Read the model definition and answer for the solid it produces. Units are mm, in the model's axes. A direction names the side the tool comes from. Coordinates: 2 decimals unless noted, no trailing zeros. Write each loop counter-clockwise with the first axis right and the second up, starting at its lowest first coordinate (ties: lowest second). Pieces come first, ordered by that corner, then holes. Notation, with made-up numbers: (-9.75, -7.5) -> (13.25, -7.5) arc R26 cw to (13.25, 15.5) -> close; hole circle Ø2 at (60, 23). An arc over 180 degrees is marked (long way). Answer in a Markdown table with one row per item. Add a question column.
Item 1: Section A-A on z = 38 is taken. Write down the section's boundary in (x, y), then the cut area to 3 significant figures.
Item 2: Section B-B on x = -20 is taken. Write down the section's boundary in (y, z).
Item 3: Straight lines are drawn through the part: line 1 (Y direction, x = -20, z = 28.8); line 2 (Y direction, x = 38, z = 28.45); line 3 (Y direction, x = 0, z = 40). For each, find the intervals that lie inside material, in ascending order. Write a range as from..to.
Item 4: Which of the six approach directions +Z, -Z, +X, -X, +Y, -Y give full straight-line access (tool end or side, diameter ignored) to faces 4 (the face through (47.35, 80.07, 37.29)), 5 (the face through (57.45, 61.37, 28.39)), 6 (the face through (10, 34, 28))?
Item 5: Given pin 1 Ø1.6 at (x, y) = (-53, 49.5) entering from +Z; pin 2 Ø1.6 at (y, z) = (34, 28) entering from -X; pin 3 Ø1 at (y, z) = (35, 29) entering from +X; pin 4 Ø10 at (x, y) = (3, 74) entering from +Z, each flat-ended and moving along its own axis, determine where each tip first touches the part or whether it passes through.
Item 6: For a pull along X with two mould halves and no side action, classify faces 1 (the face through (36.85, 40.38, 28.39)), 2 (the face through (58.718, 34.623, 28.386)), 3 (the face through (-46.7, 81.7, 45.4)) as +X half, -X half, draft (parallel to the pull), parting line (faces both ways), or undercut.
Item 7: Section C-C on y = 62 is taken. Write down the section's boundary in (x, z).
Item 8: Section D-D on x = 38 is taken. Write down the section's boundary in (y, z), then the cut area to 3 significant figures.
```python
from build123d import *

# Parameters (mm, degrees)
PAD_DEPTH     = 2
SKETCH001_R   = 3
PAD001_DEPTH  = 16
SKETCH002_R   = 1.6
SKETCH002_R_2 = 1
SKETCH002_R_3 = 1.2
SKETCH002_R_4 = 1.45
POCKET_DEPTH  = 18.001


with BuildPart() as part:
    # Sketch → Pad (new body)
    with BuildSketch(Plane.XY):
        with BuildLine():
            ThreePointArc((-50, 44), (-53.333341, 42.726773), (-54.969042, 39.555534))
            Line((-54.969042, 39.555534), (-60, -5.444466))
            ThreePointArc((-60, -5.444466), (-58.75773, -9.333341), (-55.030958, -11))
            Line((-55.030958, -11), (55.030958, -11))
            ThreePointArc((55.030958, -11), (58.75773, -9.333341), (60, -5.444466))
            Line((54.969042, 39.555534), (60, -5.444466))
            ThreePointArc((54.969042, 39.555534), (53.333341, 42.726773), (50, 44))
            Line((-50, 44), (50, 44))
        make_face()
    extrude(amount=PAD_DEPTH)

    # Sketch001 → Pad001 (join)
    with BuildSketch(Plane.XY.offset(2)):
        Circle(SKETCH001_R)
        with Locations((-48, 39)):
            Circle(SKETCH001_R)
        with Locations((48, 39)):
            Circle(SKETCH001_R)
    extrude(amount=PAD001_DEPTH)

    # Sketch002 → Pocket (cut, through all)
    with BuildSketch(Plane(origin=(0, 0, 0), x_dir=(1, 0, 0), z_dir=(0, 0, -1))):
        Circle(SKETCH002_R)
        with Locations((-48, -39)):
            Circle(SKETCH002_R)
        with Locations((48, -39)):
            Circle(SKETCH002_R)
        with Locations((9, -5.5)):
            Circle(SKETCH002_R_2)
        with Locations((9, -27)):
            Circle(SKETCH002_R_2)
        with Locations((38, 8)):
            Circle(SKETCH002_R_3)
        with Locations((38, -41)):
            Circle(SKETCH002_R_3)
        with Locations((-20, -41)):
            Circle(SKETCH002_R_3)
        with Locations((-53, -27)):
            Circle(SKETCH002_R_2)
        with Locations((-53, -5.5)):
            Circle(SKETCH002_R_2)
        with Locations((-20, 8)):
            Circle(SKETCH002_R_3)
        with Locations((-28.1, 7.74)):
            Circle(SKETCH002_R_4)
        with Locations((38, 4.5)):
            Circle(SKETCH002_R_4)
        with Locations((-28.1, -40.65)):
            Circle(SKETCH002_R_4)
        with Locations((38, -37.41)):
            Circle(SKETCH002_R_4)
        with Locations((-20, -18)):
            Circle(SKETCH002_R_3)
        with Locations((38, -18)):
            Circle(SKETCH002_R_3)
        with BuildLine():
            ThreePointArc((17, 12), (13.5, 15.5), (10, 12))
            Line((10, 12), (10, 8))
            ThreePointArc((10, 8), (13.5, 4.5), (17, 8))
            Line((17, 8), (17, 12))
        make_face()
    extrude(amount=-POCKET_DEPTH, mode=Mode.SUBTRACT)


with BuildPart() as part_1:
    # Body placement: moved
    add(part.part.moved(Location((0, 44, 27.4))))


solid = part_1.part
```
Results below:
| question | item | result |
|---|---|---|
| 1 | outline | circle Ø6 at (-48, 83); circle Ø6 at (0, 44); circle Ø6 at (48, 83); hole circle Ø3.2 at (-48, 83); hole circle Ø3.2 at (0, 44); hole circle Ø3.2 at (48, 83) |
| 1 | area | 60.7 mm2 |
| 2 | outline | (33, 27.4) -> (34.8, 27.4) -> (34.8, 29.4) -> (33, 29.4) -> close; (37.2, 27.4) -> (60.8, 27.4) -> (60.8, 29.4) -> (37.2, 29.4) -> close; (63.2, 27.4) -> (83.8, 27.4) -> (83.8, 29.4) -> (63.2, 29.4) -> close; (86.2, 27.4) -> (88, 27.4) -> (88, 29.4) -> (86.2, 29.4) -> close |
| 3 | line 1 | y = 33..34.8, 37.2..60.8, 63.2..83.8, 86.2..88 |
| 3 | line 2 | y = 33..34.8, 37.2..38.05, 40.95..60.8, 63.2..79.96, 82.86..83.8, 86.2..88 |
| 3 | line 3 | y = 41..42.4, 45.6..47 |
| 4 | face 4 | +Z |
| 4 | face 5 | +Z, -Z, +X, +Y |
| 4 | face 6 | +Z, -Z, -Y |
| 5 | pin 1 | passes through |
| 5 | pin 2 | stops at x = -58.87 |
| 5 | pin 3 | stops at x = 59.36 |
| 5 | pin 4 | stops at z = 29.4 |
| 6 | face 1 | undercut |
| 6 | face 2 | +X half |
| 6 | face 3 | draft |
| 7 | outline | (-57.38, 27.4) -> (-21.2, 27.4) -> (-21.2, 29.4) -> (-57.38, 29.4) -> close; (-18.8, 27.4) -> (36.8, 27.4) -> (36.8, 29.4) -> (-18.8, 29.4) -> close; (39.2, 27.4) -> (57.38, 27.4) -> (57.38, 29.4) -> (39.2, 29.4) -> close |
| 8 | outline | (33, 27.4) -> (34.8, 27.4) -> (34.8, 29.4) -> (33, 29.4) -> close; (37.2, 27.4) -> (38.05, 27.4) -> (38.05, 29.4) -> (37.2, 29.4) -> close; (40.95, 27.4) -> (60.8, 27.4) -> (60.8, 29.4) -> (40.95, 29.4) -> close; (63.2, 27.4) -> (79.96, 27.4) -> (79.96, 29.4) -> (63.2, 29.4) -> close; (82.86, 27.4) -> (83.8, 27.4) -> (83.8, 29.4) -> (82.86, 29.4) -> close; (86.2, 27.4) -> (88, 27.4) -> (88, 29.4) -> (86.2, 29.4) -> close |
| 8 | area | 84.0 mm2 |
